Could you check a few things on this model? Use its own coordinates, in mm. A direction names the side the tool comes from. Round coordinates to 2 decimals unless told otherwise and drop trailing zeros. Loops run counter-clockwise (first coordinate to the right, second up) from the corner with the lowest first, then second, coordinate; pieces in that order, holes last. Notation, with made-up numbers: M 9.25,53 L 20.25,53 A26 ccw 20.25,69 Z; hole C -39.75,75.25 d6. An arc over 180 degrees is marked long. Answer in a Markdown table with one row per item.
```python
from build123d import *
from OCP.BRepAlgoAPI import BRepAlgoAPI_Cut
from OCP.TopTools import TopTools_ListOfShape

# Parameters (mm, degrees)
SKETCH1_W           = 200
SKETCH1_H           = 135
BOSS_EXTRUDE1_DEPTH = 40
CUT_EXTRUDE2_DEPTH  = 40
CUT_EXTRUDE3_DEPTH  = 35
CUT_EXTRUDE4_DEPTH  = 5
CUT_EXTRUDE5_DEPTH  = 28.2
SKETCH10_W          = 2
SKETCH10_H          = 2
SKETCH10_W_2        = 15
BOSS_EXTRUDE2_DEPTH = 35
CUT_EXTRUDE6_DEPTH  = 35
SKETCH15_R          = 2
CUT_EXTRUDE8_DEPTH  = 35
CIRPATTERN1_COUNT   = 4
SKETCH16_R          = 2.5
CUT_EXTRUDE9_DEPTH  = 35
SKETCH17_R          = 30.2
CUT_EXTRUDE10_DEPTH = 38
BOSS_EXTRUDE3_DEPTH = 34
SKETCH19_R          = 28.43
CUT_EXTRUDE11_DEPTH = 41
SKETCH20_R          = 51
CUT_EXTRUDE12_DEPTH = 30
SCALE6_SCALE        = 1.33
SKETCH23_R          = 15
CUT_EXTRUDE15_DEPTH = 252.625115321


with BuildPart() as part:
    # Sketch1 → Boss-Extrude1 (new body)
    with BuildSketch(Plane.XY):
        with Locations((100, 67.5)):
            Rectangle(SKETCH1_W, SKETCH1_H)
    extrude(amount=BOSS_EXTRUDE1_DEPTH)

    # Sketch6 → Cut-Extrude2 (cut)
    with BuildSketch(Plane.XY.offset(40)):
        with BuildLine():
            Line((0, 62.5), (37.5, 62.5))
            ThreePointArc((37.5, 62.5), (43.403842887, 89.016504294), (60, 110.523431781))
            Line((60, 110.523431781), (60, 135))
            Line((60, 135), (0, 135))
            Line((0, 135), (0, 62.5))
        make_face()
        with BuildLine():
            Line((0, 0), (100, 0))
            ThreePointArc((100, 0), (55.805826176, 18.305826176), (37.5, 62.5))
            Line((37.5, 62.5), (0, 62.5))
            Line((0, 62.5), (0, 0))
        make_face()
        with BuildLine():
            ThreePointArc((162.5, 62.5), (144.194173824, 18.305826176), (100, 0))
            Line((100, 0), (200, 0))
            Line((200, 0), (200, 135))
            Line((200, 135), (140, 135))
            Line((140, 135), (140, 110.523431781))
            ThreePointArc((140, 110.523431781), (156.596157113, 89.016504294), (162.5, 62.5))
        make_face()
    extrude(amount=-CUT_EXTRUDE2_DEPTH, mode=Mode.SUBTRACT)

    # Sketch7 → Cut-Extrude3 (cut)
    with BuildSketch(Plane.XY.offset(40)):
        with BuildLine():
            ThreePointArc((155, 62.5), (79.689903988, 11.387379249), (60, 100.249172176))
            Line((60, 100.249172176), (60, 110.523431781))
            ThreePointArc((60, 110.523431781), (100, 0), (140, 110.523431781))
            Line((140, 110.523431781), (140, 100.249172176))
            ThreePointArc((140, 100.249172176), (151.112620751, 82.810096012), (155, 62.5))
        make_face()
    extrude(amount=-CUT_EXTRUDE3_DEPTH, mode=Mode.SUBTRACT)

    # Sketch8 → Cut-Extrude4 (cut)
    with BuildSketch(Plane.XY.offset(40)):
        with BuildLine():
            Line((60, 135), (60, 100.249172176))
            ThreePointArc((60, 100.249172176), (100, 117.5), (140, 100.249172176))
            Line((140, 100.249172176), (140, 135))
            Line((140, 135), (60, 135))
        make_face()
    extrude(amount=-CUT_EXTRUDE4_DEPTH, mode=Mode.SUBTRACT)

    # Sketch9 → Cut-Extrude5 (cut)
    with BuildSketch(Plane(origin=(0, 0, 0), x_dir=(-1, 0, 0), z_dir=(0, 0, -1))):
        with BuildLine():
            Line((-71.8, 62.5), (-100, 62.5))
            Line((-100, 62.5), (-128.2, 62.5))
            Line((-128.2, 62.5), (-128.2, 103.788739385))
            ThreePointArc((-128.2, 103.788739385), (-123.34523506, 18.284618061), (-50, 62.5))
            ThreePointArc((-50, 62.5), (-55.784618061, 85.84523506), (-71.8, 103.788739385))
            Line((-71.8, 103.788739385), (-71.8, 62.5))
        make_face()
        with BuildLine():
            Line((-128.2, 62.5), (-100, 62.5))
            Line((-100, 62.5), (-100, 112.5))
            ThreePointArc((-100, 112.5), (-114.757422383, 110.272570421), (-128.2, 103.788739385))
            Line((-128.2, 103.788739385), (-128.2, 62.5))
        make_face()
        with BuildLine():
            Line((-100, 112.5), (-100, 62.5))
            Line((-100, 62.5), (-71.8, 62.5))
            Line((-71.8, 62.5), (-71.8, 103.788739385))
            ThreePointArc((-71.8, 103.788739385), (-85.242577617, 110.272570421), (-100, 112.5))
        make_face()
    extrude(amount=-CUT_EXTRUDE5_DEPTH, mode=Mode.SUBTRACT)

    # Sketch10 → Boss-Extrude2 (add)
    with BuildSketch(Plane.XY.offset(40)):
        with Locations((154, 1)):
            Rectangle(SKETCH10_W, SKETCH10_H)
        with Locations((162.5, 1)):
            Rectangle(SKETCH10_W_2, SKETCH10_H)
        with BuildLine():
            Line((155, 2), (155, 62.5))
            ThreePointArc((155, 62.5), (154.497706374, 55.083801513), (153, 47.803061543))
            Line((153, 47.803061543), (153, 2))
            Line((153, 2), (155, 2))
        make_face()
        with BuildLine():
            ThreePointArc((47, 47.803061543), (45.502293626, 55.083801513), (45, 62.5))
            Line((45, 62.5), (45, 2))
            Line((45, 2), (30, 2))
            Line((30, 2), (30, 0))
            Line((30, 0), (47, 0))
            Line((47, 0), (47, 47.803061543))
        make_face()
    extrude(amount=-BOSS_EXTRUDE2_DEPTH)

    # Sketch12 → Cut-Extrude6 (cut)
    with BuildSketch(Plane(origin=(0, 135, 0), x_dir=(1, 0, 0), z_dir=(0, 1, 0))):
        with BuildLine():
            Line((100, 0), (71.8, 0))
            ThreePointArc((71.8, 0), (73.365155008, -9.264180065), (77.886881721, -17.5))
            Line((77.886881721, -17.5), (100, -17.5))
            Line((100, -17.5), (100, 0))
        make_face()
        with BuildLine():
            Line((128.2, 0), (100, 0))
            Line((100, 0), (100, -17.5))
            Line((100, -17.5), (77.886881721, -17.5))
            ThreePointArc((77.886881721, -17.5), (109.264180065, -26.634844992), (128.2, 0))
        make_face()
    extrude(amount=-CUT_EXTRUDE6_DEPTH, mode=Mode.SUBTRACT)

    # Sketch15 → Cut-Extrude8 (cut)
    with BuildSketch(Plane(origin=(0, 0, 0), x_dir=(-1, 0, 0), z_dir=(0, 0, -1))):
        with Locations((-41.25, 62.5)):
            Circle(SKETCH15_R)
    cut_extrude8 = extrude(amount=-CUT_EXTRUDE8_DEPTH, mode=Mode.SUBTRACT)

    # CirPattern1: Cut-Extrude8 ×4 about axis
    cirpattern1_axis = Axis((100, 62.5, 0), (0, 0, 1))
    for i in range(1, CIRPATTERN1_COUNT):
        add(cut_extrude8.rotate(cirpattern1_axis, i * 360 / CIRPATTERN1_COUNT), mode=Mode.SUBTRACT)

    # Sketch16 → Cut-Extrude9 (cut)
    with BuildSketch(Plane(origin=(0, 2, 0), x_dir=(1, 0, 0), z_dir=(0, 1, 0))):
        with Locations(Location((162.5, -22.5, 0), (0, 0, 180))):
            Circle(SKETCH16_R)
        with Locations(Location((37.5, -22.5, 0), (0, 0, 180))):
            Circle(SKETCH16_R)
    extrude(amount=-CUT_EXTRUDE9_DEPTH, mode=Mode.SUBTRACT)

    # Sketch17 → Cut-Extrude10 (cut)
    with BuildSketch(Plane(origin=(0, 135, 0), x_dir=(1, 0, 0), z_dir=(0, 1, 0))):
        with Locations((100, 0)):
            Circle(SKETCH17_R)
    extrude(amount=-CUT_EXTRUDE10_DEPTH, mode=Mode.SUBTRACT)

    # Sketch18 → Boss-Extrude3 (add)
    with BuildSketch(Plane(origin=(0, 135, 0), x_dir=(1, 0, 0), z_dir=(0, 1, 0))):
        with BuildLine():
            Line((130.2, 0), (69.8, 0))
            ThreePointArc((69.8, 0), (100, -30.2), (130.2, 0))
        make_face()
    extrude(amount=-BOSS_EXTRUDE3_DEPTH)

    # Sketch19 → Cut-Extrude11 (cut)
    with BuildSketch(Plane(origin=(0, 135, 0), x_dir=(1, 0, 0), z_dir=(0, 1, 0))):
        with Locations((100, 0)):
            Circle(SKETCH19_R)
    extrude(amount=-CUT_EXTRUDE11_DEPTH, mode=Mode.SUBTRACT)

    # Sketch20 → Cut-Extrude12 (cut)
    with BuildSketch(Plane(origin=(0, 0, 0), x_dir=(-1, 0, 0), z_dir=(0, 0, -1))):
        with Locations((-100, 62.5)):
            Circle(SKETCH20_R)
    extrude(amount=-CUT_EXTRUDE12_DEPTH, mode=Mode.SUBTRACT)


with BuildPart() as part_1:
    # Scale6: scaled about (99.999974062, 70.397501242, 26.101442842)
    add(part.part.scale(SCALE6_SCALE).moved(Location((-32.99999144, -23.23117541, -8.613476138))))


with BuildPart() as cut_extrude15_tool:
    # Sketch23 → Cut-Extrude15 (new, through all)
    with BuildSketch(Plane(origin=(0, 0, 31.286528804), x_dir=(-1, 0, 0), z_dir=(0, 0, -1))):
        with Locations((-100.069201604, 59.906371454)):
            Circle(SKETCH23_R)
    extrude(amount=-CUT_EXTRUDE15_DEPTH)


with BuildPart() as part_2:
    add(part_1.part)

    # Cut-Extrude15: cut by cut_extrude15_tool, with a tolerance
    cut_extrude15_stock = TopTools_ListOfShape()
    cut_extrude15_stock.Append(part_2.part.wrapped)
    cut_extrude15_tools = TopTools_ListOfShape()
    cut_extrude15_tools.Append(cut_extrude15_tool.part.wrapped)
    cut_extrude15_cut = BRepAlgoAPI_Cut()
    cut_extrude15_cut.SetArguments(cut_extrude15_stock)
    cut_extrude15_cut.SetTools(cut_extrude15_tools)
    cut_extrude15_cut.SetFuzzyValue(0.00001)
    cut_extrude15_cut.Build()
    add(Compound.cast(cut_extrude15_cut.Shape()).solids(), mode=Mode.REPLACE)


solid = part_2.part
```
1) I want a section at D-D, the plane x = 55.5. Please give me the cut outline in (y, z).
Computed:
| item | result |
|---|---|
| outline | M -10.32,-8.61 L 8.7,-8.61 L 8.7,31.29 L 111.09,31.29 L 111.09,-8.61 L 156.32,-8.61 L 156.32,37.94 L 117.95,37.94 L 117.95,44.59 L 1.84,44.59 L 1.84,-1.96 L -10.32,-1.96 Z |
2) I want a section at B-B, the plane x = 109. Please give me the cut outline in (y, z), plus the area to 3 significant figures.
Computed:
| item | result |
|---|---|
| outline | M -22.74,-8.61 L -7.34,-8.61 L -7.34,31.29 L 47.85,31.29 L 47.85,44.59 L -12.7,44.59 L -12.7,-1.96 L -22.74,-1.96 Z; M 71.96,31.29 L 127.12,31.29 L 127.12,28.11 L 156.32,28.11 L 156.32,37.94 L 132.49,37.94 L 132.49,44.59 L 71.96,44.59 Z |
| area | 2,140 mm² |
3) Which directions (+Z, -Z, +X, -X, +Y, -Y) give clear straight access to the entire face, cutting with the end or side of a thin tool? Please do faces 1 (the face through (26.85, 20, 22)), 2 (the face through (114.704, -6.323, 11.057)), 3 (the face through (100, -15, -1.963)), 4 (the face through (188, -20.571, 22)), 5 (the face through (13, -20.571, 22)).
Computed:
| item | result |
|---|---|
| face 1 | +Z, -X, +Y |
| face 2 | -Z |
| face 3 | +Z, -Y |
| face 4 | +Z, -Z, +X, +Y |
| face 5 | +Z, -Z, -X, +Y |
4) If we mould it in two halves opening along Z, with no side actions, what happens to faces 6 (the face through (19.326, -21.883, 23.559)), 7 (the face through (119, 56, 44.587)), 8 (the face through (46.8, 133, 15))? For each: released by +Z, released by -Z, zero draft, split by the parting line, or undercut.
Computed:
| item | result |
|---|---|
| face 6 | undercut |
| face 7 | released by +Z |
| face 8 | zero draft |
5) I want a section at C-C, the plane z = 12. Please give me the cut outline in (x, y), plus the area to 3 significant figures.
Computed:
| item | result |
|---|---|
| outline | M 6.9,-23.23 L 29.51,-23.23 L 29.51,40.35 A73.15 ccw 170.49,40.35 L 170.49,-23.23 L 193.1,-23.23 L 193.1,-20.57 L 173.15,-20.57 L 173.15,59.89 A73.15 ccw 153.2,110.1 L 153.2,156.32 L 131.7,156.32 L 131.7,119.86 A67.83 cw long 68.3,119.86 L 68.3,156.32 L 46.8,156.32 L 46.8,110.1 A73.15 ccw 26.85,59.89 L 26.85,-20.57 L 6.9,-20.57 Z |
| area | 4,090 mm² |
6) I need wall thicknesses on line 1 (X direction, y = -2, z = 30.5); line 2 (Z direction, x = 77, y = 18); line 3 (X direction, y = 27, z = -2.5). Which ranges of each line are inside material? Lowest first, please.
Computed:
| item | result |
|---|---|
| line 1 | x = 26.85 to 29.51, 61.01 to 72.25, 127.75 to 138.99, 170.49 to 173.15 |
| line 2 | z = 31.29 to 44.59 |
| line 3 | x = 23.66 to 40.68, 159.32 to 176.34 |
7) I want a section at A-A, the plane y = 71. Please give me the cut outline in (x, z), plus the area to 3 significant figures.
Computed:
| item | result |
|---|---|
| outline | M 17.62,-8.61 L 33.09,-8.61 L 33.09,31.29 L 89.97,31.29 L 89.97,44.59 L 27.7,44.59 L 27.7,-1.96 L 17.62,-1.96 Z; M 110.17,31.29 L 166.91,31.29 L 166.91,-8.61 L 182.38,-8.61 L 182.38,-1.96 L 172.3,-1.96 L 172.3,44.59 L 110.17,44.59 Z |
| area | 2,220 mm² |
8) Will these pins go through, and if not, where does the flat tip stop? P1, Ø7, axis at x = 100, y = -18.24, coming from the -Z side; P2, Ø5, axis at x = 178.14, y = 59.89, coming from the -Z side; P3, Ø12, axis at y = 75, z = 18, coming from the +X side; P4, Ø16, axis at x = 187.5, z = 31, coming from the +Y side.
Computed:
| item | result |
|---|---|
| P1 | stops at z = -8.61 |
| P2 | passes through |
| P3 | stops at x = 172.58 |
| P4 | stops at y = -20.57 |
